Read the model definition and answer for the solid it produces. Units are mm, in the model's axes. Give positions to 0.01 mm unless a question says otherwise; leave off trailing zeros. Order: outer loops, then holes, each group sorted by start corner. A loop starts at its lowest first (then second) coordinate and runs counter-clockwise, first axis right, second up. Notation, with made-up numbers: (-30.75, -24.75) - (-12.75, -24.75) arc R16 cw to (-12.75, 2.25) - close; hole circle Ø5 at (69, -16.5). An arc over 180 degrees is marked (long way). Return JSON: item names as keys, results as strings.
```python
from build123d import *

# Parameters (mm, degrees)
SKETCH_1_W          = 300
SKETCH_1_H          = 300
EXTRUDE_1_DEPTH     = 10
SKETCH_2_R          = 20
CUT_EXTRUDE_1_DEPTH = 213.367605816
SKETCH_5_W          = 300
SKETCH_5_H          = 10
EXTRUDE_2_DEPTH     = 25
SKETCH_7_R          = 2.5
CUT_EXTRUDE_5_DEPTH = 231.705439901


with BuildPart() as part:
    # 草图1 → 凸台-拉伸1 (new body)
    with BuildSketch(Plane.XY):
        Rectangle(SKETCH_1_W, SKETCH_1_H)
    extrude(amount=EXTRUDE_1_DEPTH)

    # 草图2 → 切除-拉伸1 (cut, through all)
    with BuildSketch(Plane.XY.offset(10)):
        with Locations((-70, -70)):
            Circle(SKETCH_2_R)
        with Locations((71.421356237, -20)):
            Circle(SKETCH_2_R)
        with Locations((-24.625507324, 60)):
            Circle(SKETCH_2_R)
        with Locations((71.421356237, 25)):
            Circle(SKETCH_2_R)
    extrude(amount=-CUT_EXTRUDE_1_DEPTH, mode=Mode.SUBTRACT)

    # 草图5 → 凸台-拉伸2 (add)
    with BuildSketch(Plane.XZ.offset(150)):
        with Locations((0, 5)):
            Rectangle(SKETCH_5_W, SKETCH_5_H)
    extrude(amount=EXTRUDE_2_DEPTH)

    # 草图7 → 切除-拉伸5 (cut, through all)
    with BuildSketch(Plane(origin=(0, 0, 0), x_dir=(-1, 0, 0), z_dir=(0, 0, -1))):
        with Locations((129.453643763, -143.875)):
            Circle(SKETCH_7_R)
        with Locations((102.453643763, -143.875)):
            Circle(SKETCH_7_R)
        with Locations((129.453643763, -170.875)):
            Circle(SKETCH_7_R)
        with Locations((102.453643763, -170.875)):
            Circle(SKETCH_7_R)
    extrude(amount=-CUT_EXTRUDE_5_DEPTH, mode=Mode.SUBTRACT)


solid = part.part
```
Q1. Consider L1, parallel to X at y = -144.5, z = 5.75; L2, parallel to Y at x = 78, z = 3.25; L3, parallel to Y at x = 85, z = 2.5. Determine where each line is inside the solid, lowest interval first.
Values:
{"L1": "x = -150 to -131.87, -127.03 to -104.87, -100.03 to 150", "L2": "y = -175 to -38.89, -1.11 to 6.11, 43.89 to 150", "L3": "y = -175 to -34.68, -5.32 to 10.32, 39.68 to 150"}
Q2. A cutting plane is placed at C-C (x = 62). Write down the section's boundary in (y, z).
Values:
{"outline": "(-175, 0) - (-37.64, 0) - (-37.64, 10) - (-175, 10) - close; (-2.36, 0) - (7.36, 0) - (7.36, 10) - (-2.36, 10) - close; (42.64, 0) - (150, 0) - (150, 10) - (42.64, 10) - close"}
Q3. A cutting plane is placed at D-D (z = 4.25). Give the number of separate pieces and of enclosed holes in the cut face, and give its area (3 significant figures).
Values:
{"separate pieces": "1", "enclosed holes": "8", "area": "92,400 mm²"}
Q4. Determine the mould class of faces 1 (the flat face through (-2, -175, 5)), 2 (the flat face through (-150, -10, 5)), 3 (the cylindrical face through (89.896, 17.34, 5.07)), 4 (the cylindrical face through (90.5, -14, 5.1)) for opening direction X: released by +X, released by -X, zero draft, split by the parting line, or undercut.
Values:
{"face 1": "zero draft", "face 2": "released by -X", "face 3": "undercut", "face 4": "undercut"}
Q5. Given pin 1 (4.5 mm diameter, centred on x = -129.45, y = -170.88, fed in from +Z), flat-ended and moving along its own axis, determine where the tip first touches the part or whether it passes through.
Values:
{"pin 1": "passes through"}
Q6. A cutting plane is placed at B-B (x = -70). Write down the section's boundary in (y, z).
Values:
{"outline": "(-175, 0) - (-90, 0) - (-90, 10) - (-175, 10) - close; (-50, 0) - (150, 0) - (150, 10) - (-50, 10) - close"}
Q7. A cutting plane is placed at A-A (y = 25). Write down the section's boundary in (x, z), and give its area (3 significant figures).
Values:
{"outline": "(-150, 0) - (51.42, 0) - (51.42, 10) - (-150, 10) - close; (91.42, 0) - (150, 0) - (150, 10) - (91.42, 10) - close", "area": "2,600 mm²"}
